Geometry: final body of the model. Coordinates: model frame, mm. Round coordinates to 2 decimals unless told otherwise and drop trailing zeros. Loops run counter-clockwise (first coordinate to the right, second up) from the corner with the lowest first, then second, coordinate; pieces in that order, holes last. Notation, with made-up numbers: (38, 34) - (87, 34) arc R9 cw to (87, 48) - close; hole circle Ø11 at (-4.75, 7). An arc over 180 degrees is marked (long way). Write item = value, one per line. Start each with the question number.
Item 1: Section B-B (x = 0). Return loops of the section in (y, z) (3 decimals).
Item 2: Section A-A (y = -1). Return loops of the section in (x, z) (3 decimals).
Item 3: Line query: line 1 (X direction, y = -2.6, z = 0) (3 decimals); line 2 (Y direction, x = -19, z = -13); line 3 (Z direction, x = -15.5, y = -1.85). Output: solid intervals per line, ascending. Write a range as from..to.
Item 4: First-contact query: pin 1 (0.5 mm diameter, centred on y = -0.5, z = 25, fed in from +X); pin 2 (0.5 mm diameter, centred on y = -1, z = -25.5, fed in from -X); pin 3 (0.6 mm diameter, centred on x = 25.5, z = -1.5, fed in from +Y); pin 4 (2 mm diameter, centred on x = 11.5, z = 15.5, fed in from -Y). Flat tips, straight axial feed; report the tip coordinate or a pass-through.
Item 5: Section C-C (z = 0). Return loops of the section in (x, y) (3 decimals).
Item 6: Section D-D (x = 9). Return loops of the section in (y, z) (3 decimals), plus the area to 3 significant figures.
from build123d import *

# Parameters (mm, degrees)
SKETCH1_R            = 28.575
SHAFT_DEPTH          = 4.445
SKETCH11_R           = 22.225
THRU_HOLE_DEPTH      = 41.654880088
TOOLING_POINTS_DEPTH = 1.651
RETAINER_START       = -2.667
SKETCH12_R           = 24.765
RETAINER_HOLE_DEPTH  = 2.667


with BuildPart() as part:
    # Sketch1 → Shaft (new body)
    with BuildSketch(Plane(origin=(0, 0, 0), x_dir=(1, 0, 0), z_dir=(0, 1, 0))):
        with Locations(Location((0, 0, 0), (0, 0, 270))):
            Circle(SKETCH1_R)
    extrude(amount=-SHAFT_DEPTH)

    # Sketch11 → Thru Hole (cut, through all)
    with BuildSketch(Plane(origin=(0, 0, 0), x_dir=(-1, 0, 0), z_dir=(0, 1, 0))):
        with Locations(Location((0, 0, 0), (0, 0, 90))):
            Circle(SKETCH11_R)
    extrude(amount=-THRU_HOLE_DEPTH, mode=Mode.SUBTRACT)

    # Sketch13 → Tooling Points (cut)
    with BuildSketch(Plane(origin=(0, 0, 0), x_dir=(-1, 0, 0), z_dir=(0, 1, 0))):
        with BuildLine():
            Line((-24.470168062, -3.81), (-26.268131814, -3.81))
            ThreePointArc((-26.268131814, -3.81), (-26.543, 0), (-26.268131814, 3.81))
            Line((-26.268131814, 3.81), (-24.470168062, 3.81))
            ThreePointArc((-24.470168062, 3.81), (-24.765, 0), (-24.470168062, -3.81))
        make_face()
        with BuildLine():
            Line((3.81, -24.470168062), (3.81, -26.268131814))
            ThreePointArc((3.81, -26.268131814), (0, -26.543), (-3.81, -26.268131814))
            Line((-3.81, -26.268131814), (-3.81, -24.470168062))
            ThreePointArc((-3.81, -24.470168062), (0, -24.765), (3.81, -24.470168062))
        make_face()
        with BuildLine():
            Line((24.470168062, 3.81), (26.268131814, 3.81))
            ThreePointArc((26.268131814, 3.81), (26.543, 0), (26.268131814, -3.81))
            Line((26.268131814, -3.81), (24.470168062, -3.81))
            ThreePointArc((24.470168062, -3.81), (24.765, 0), (24.470168062, 3.81))
        make_face()
        with BuildLine():
            Line((-3.81, 24.470168062), (-3.81, 26.268131814))
            ThreePointArc((-3.81, 26.268131814), (0, 26.543), (3.81, 26.268131814))
            Line((3.81, 26.268131814), (3.81, 24.470168062))
            ThreePointArc((3.81, 24.470168062), (0, 24.765), (-3.81, 24.470168062))
        make_face()
    extrude(amount=-TOOLING_POINTS_DEPTH, mode=Mode.SUBTRACT)

    # Sketch12 → Retainer Hole (cut)
    with BuildSketch(Plane.XZ.offset(4.445).offset(RETAINER_START)):
        with Locations(Location((0, 0, 0), (0, 0, 270))):
            Circle(SKETCH12_R)
    extrude(amount=RETAINER_HOLE_DEPTH, mode=Mode.SUBTRACT)


solid = part.part
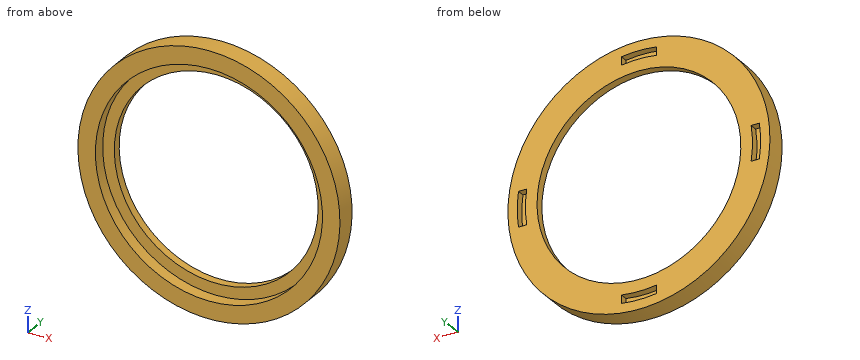
Taken from the geometry:
q1.outline = (-4.445, -28.575) - (0, -28.575) - (0, -26.543) - (-1.651, -26.543) - (-1.651, -24.765) - (0, -24.765) - (0, -22.225) - (-1.778, -22.225) - (-1.778, -24.765) - (-4.445, -24.765) - close; (-4.445, 24.765) - (-1.778, 24.765) - (-1.778, 22.225) - (0, 22.225) - (0, 24.765) - (-1.651, 24.765) - (-1.651, 26.543) - (0, 26.543) - (0, 28.575) - (-4.445, 28.575) - close
q2.outline = circle Ø57.15 at (0, 0); hole (-26.268, -3.81) - (-24.47, -3.81) arc R24.765 cw to (-24.47, 3.81) - (-26.268, 3.81) arc R26.543 ccw to start; hole circle Ø44.45 at (0, 0); hole (-3.81, -26.268) arc R26.543 ccw to (3.81, -26.268) - (3.81, -24.47) arc R24.765 cw to (-3.81, -24.47) - close; hole (-3.81, 24.47) arc R24.765 cw to (3.81, 24.47) - (3.81, 26.268) arc R26.543 ccw to (-3.81, 26.268) - close; hole (24.47, -3.81) - (26.268, -3.81) arc R26.543 ccw to (26.268, 3.81) - (24.47, 3.81) arc R24.765 cw to start
q3.line_1 = -28.575..-24.765, 24.765..28.575
q3.line_2 = -1.78..0
q3.line_3 = -24.01..-19.31, 19.31..24.01
q4.pin_1 = 14.28
q4.pin_2 = -13.38
q4.pin_3 = -1.65
q4.pin_4 = through
q5.outline = (-28.575, -4.445) - (-24.765, -4.445) - (-24.765, -1.778) - (-22.225, -1.778) - (-22.225, 0) - (-24.765, 0) - (-24.765, -1.651) - (-26.543, -1.651) - (-26.543, 0) - (-28.575, 0) - close; (22.225, -1.778) - (24.765, -1.778) - (24.765, -4.445) - (28.575, -4.445) - (28.575, 0) - (26.543, 0) - (26.543, -1.651) - (24.765, -1.651) - (24.765, 0) - (22.225, 0) - close
q6.outline = (-4.445, -27.121) - (0, -27.121) - (0, -20.321) - (-1.778, -20.321) - (-1.778, -23.072) - (-4.445, -23.072) - close; (-4.445, 23.072) - (-1.778, 23.072) - (-1.778, 20.321) - (0, 20.321) - (0, 27.121) - (-4.445, 27.121) - close
q6.area = 45.8 mm^2
